from build123d import *

# Parameters (mm, degrees)
F0_W     = 6.35
F0_H     = 6.35
F0_R     = 1.905
F1_DEPTH = 25.4
F0_R_2   = 5.08
F2_DEPTH = 12.7
F3_DEPTH = 38.1


with BuildPart() as f1:
    # F0 (on Top) → F1 (new body)
    with BuildSketch(Plane.XY):
        with BuildLine():
            Line((-57.149317, -33.320757), (-32.990752, -33.320757))
            Line((-32.990752, -33.320757), (-32.990752, -26.970757))
            Line((-32.990752, -26.970757), (-53.74143, -26.970757))
            ThreePointArc((-53.74143, -26.970757), (-54.64724, -30.574096), (-57.149317, -33.320757))
        make_face()
        with Locations((-29.815752, -30.145757)):
            Rectangle(F0_W, F0_H)
        with Locations((-29.815752, -30.145757)):
            Circle(F0_R, mode=Mode.SUBTRACT)
        with Locations((-23.465752, -30.145757)):
            Rectangle(F0_W, F0_H)
        with Locations((-23.465752, -30.145757)):
            Circle(F0_R, mode=Mode.SUBTRACT)
    extrude(amount=-F1_DEPTH)

    # F0 (on Top) → F2 (join)
    with BuildSketch(Plane.XY):
        with BuildLine():
            ThreePointArc((-57.149317, -20.620757), (-68.98143, -26.970757), (-57.149317, -33.320757))
            ThreePointArc((-57.149317, -33.320757), (-54.64724, -30.574096), (-53.74143, -26.970757))
            ThreePointArc((-53.74143, -26.970757), (-54.64724, -23.367419), (-57.149317, -20.620757))
        make_face()
        with Locations((-61.36143, -26.970757)):
            Circle(F0_R_2, mode=Mode.SUBTRACT)
    extrude(amount=-F2_DEPTH)

    # F0 (on Top) → F3 (join)
    with BuildSketch(Plane.XY):
        with BuildLine():
            Line((-57.149317, -33.320757), (-32.990752, -33.320757))
            Line((-32.990752, -33.320757), (-32.990752, -26.970757))
            Line((-32.990752, -26.970757), (-53.74143, -26.970757))
            ThreePointArc((-53.74143, -26.970757), (-54.64724, -30.574096), (-57.149317, -33.320757))
        make_face()
    extrude(amount=F3_DEPTH)

    # F4: F1 across face


with BuildPart() as f1_1:
    add(f1.part)
    add(f1.part.mirror(Plane(origin=(-43.892507, -30.223136, 38.1), x_dir=(1, 0, 0), z_dir=(0, 0, 1))))


solid = f1_1.part
Work out the finished part from the listing and answer in its coordinate system (mm). A direction names the side the tool comes from. Give positions to 0.01 mm unless a question says otherwise; leave off trailing zeros. Write each loop counter-clockwise with the first axis right and the second up, starting at its lowest first coordinate (ties: lowest second). Pieces come first, ordered by that corner, then holes. Notation, with made-up numbers: (-31.75, 82) - (8.25, 82) arc R23 cw to (8.25, 115) - close; hole circle Ø10 at (-23, -10). An arc over 180 degrees is marked (long way). One line per item, written item: value. Start each with the question number.
1. Consider probe 1 along Z at (x, y) = (-32.5, -31.25); probe 2 along Y at (x, z) = (-38, 56.5); probe 3 along Y at (x, z) = (-28.5, -2.5). Determine where each line is inside the solid, lowest interval first.
2. Given pin 1 (11 mm diameter, centred on x = -35, z = 36, fed in from -Y); pin 2 (7.5 mm diameter, centred on x = -65, y = -27.5, fed in from +Z); pin 3 (8 mm diameter, centred on x = -61.36, y = -26.97, fed in from -Z); pin 4 (3 mm diameter, centred on y = -29.5, z = 41.5, fed in from +X), each flat-ended and moving along its own axis, determine where each tip first touches the part or whether it passes through.
3. Find section C-C (y = -25). Write down the section's boundary in (x, z), then the cut area to 3 significant figures.
4. Find section B-B (z = 92). Write down the section's boundary in (x, y) (3 decimals).
5. Find section A-A (x = -29.5). Write down the section's boundary in (y, z), then the cut area to 3 significant figures.
6. Find section D-D (z = 75). Write down the section's boundary in (x, y).
7. For a pull along Y with two mould halves and no side action, classify faces 1 (the flat face through (-27, -30, 76.2)), 2 (the flat face through (-43, -33.321, 39)), 3 (the cylindrical face through (-28.937, -31.836, 88.722)) as +Y half, -Y half, draft (parallel to the pull), parting line (faces both ways), or undercut.
8. For faces 4 (the flat face through (-32.991, -30, 39)), 5 (the flat face through (-56, -29, -12.7)), 6 (the flat face through (-40, -26.971, 39)), 7 (the flat face through (-56, -29, 0)), 8 (the flat face through (-56, -29, 88.9)), determine the directions among +Z, -Z, +X, -X, +Y, -Y from which every point of the face is accessible in a straight line to the end or side of a thin tool.
Geometry results:
1. probe 1: -25.4 to 0, 76.2 to 101.6
1. probe 2: -33.32 to -26.97
1. probe 3: -33.32 to -31.52, -28.77 to -26.97
2. pin 1: y = -33.32
2. pin 2: z = 88.9
2. pin 3: through
2. pin 4: x = -32.99
3. outline: (-68.72, -12.7) - (-66.04, -12.7) - (-66.04, 0) - (-68.72, 0) - close; (-68.72, 76.2) - (-66.04, 76.2) - (-66.04, 88.9) - (-68.72, 88.9) - close; (-56.68, -12.7) - (-54, -12.7) - (-54, 0) - (-56.68, 0) - close; (-56.68, 76.2) - (-54, 76.2) - (-54, 88.9) - (-56.68, 88.9) - close
3. area: 136 mm2
4. outline: (-57.149, -33.321) - (-20.291, -33.321) - (-20.291, -26.971) - (-53.741, -26.971) arc R7.62 cw to start; hole circle Ø3.81 at (-29.816, -30.146); hole circle Ø3.81 at (-23.466, -30.146)
5. outline: (-33.32, -25.4) - (-32.02, -25.4) - (-32.02, 0) - (-33.32, 0) - close; (-33.32, 76.2) - (-32.02, 76.2) - (-32.02, 101.6) - (-33.32, 101.6) - close; (-28.27, -25.4) - (-26.97, -25.4) - (-26.97, 0) - (-28.27, 0) - close; (-28.27, 76.2) - (-26.97, 76.2) - (-26.97, 101.6) - (-28.27, 101.6) - close
5. area: 132 mm2
6. outline: (-57.15, -33.32) - (-32.99, -33.32) - (-32.99, -26.97) - (-53.74, -26.97) arc R7.62 cw to start
7. face 1: draft
7. face 2: -Y half
7. face 3: undercut
8. face 4: +X, +Y, -Y
8. face 5: -Z, -X, +Y
8. face 6: +Z, -Z, +X, +Y
8. face 7: -X, +Y
8. face 8: +Z, -X, +Y
